Drawing for the job (mm, zero at the part's lowest x, y, z). Coordinates: 2 decimals unless noted, no trailing zeros. Loops run counter-clockwise (first coordinate to the right, second up) from the corner with the lowest first, then second, coordinate; pieces in that order, holes last. Notation, with made-up numbers: (1.5, 2) - (59.5, 2) arc R18 cw to (59.5, 21) - close; hole circle Ø11 at (22.25, 38). An arc over 180 degrees is marked (long way). One line per item, written item: value.
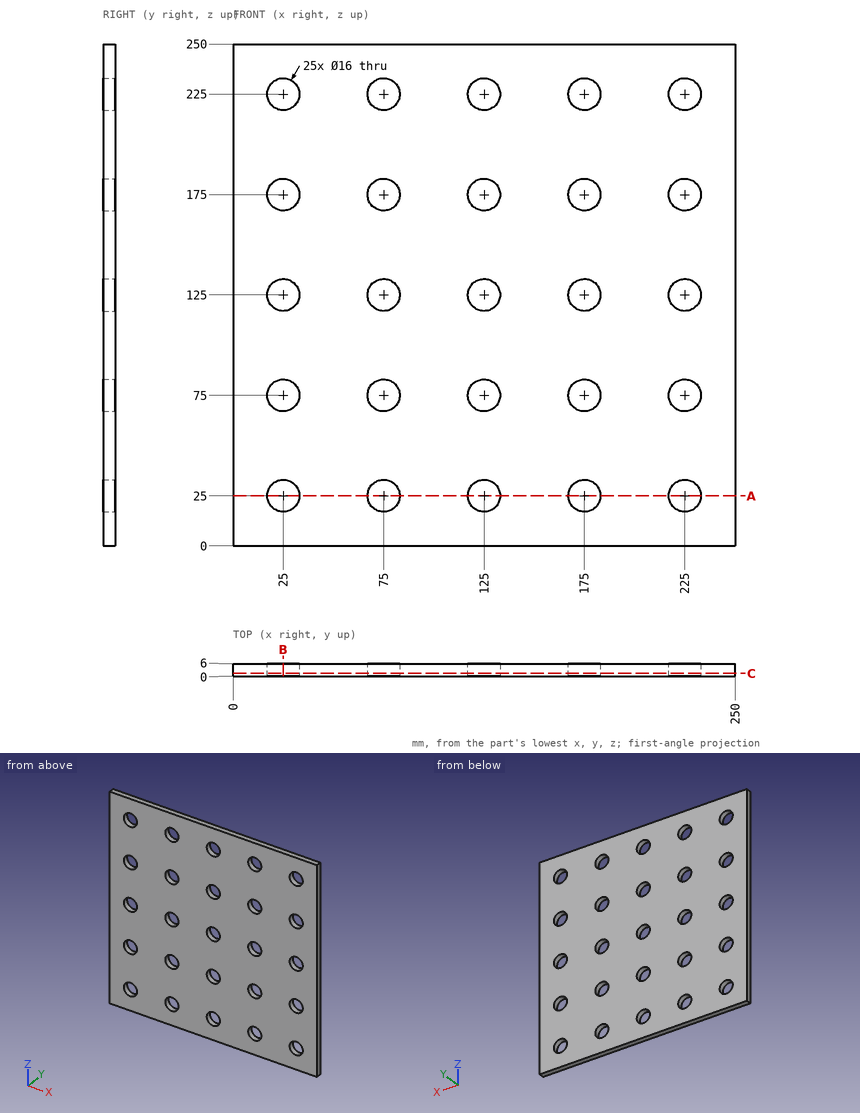
Item 1: Cut at B-B, the plane x = 25. Write the cut outline in (y, z), then the cut area to 3 significant figures.
Check result:
outline: (0, 0) - (6, 0) - (6, 17) - (0, 17) - close; (0, 33) - (6, 33) - (6, 67) - (0, 67) - close; (0, 83) - (6, 83) - (6, 117) - (0, 117) - close; (0, 133) - (6, 133) - (6, 167) - (0, 167) - close; (0, 183) - (6, 183) - (6, 217) - (0, 217) - close; (0, 233) - (6, 233) - (6, 250) - (0, 250) - close
area: 1,020 mm^2
Item 2: Cut at C-C, the plane y = 1.3. Give the number of separate pieces and of enclosed holes in the cut face, then the cut area to 3 significant figures.
Check result:
separate pieces: 1
enclosed holes: 25
area: 57,500 mm^2
Item 3: Probe probe 1 along Z at (x, y) = (225, 2.9); probe 2 along Z at (x, y) = (81.5, 1). List the from-to ranges inside material, lowest first. Write a range as from..to.
Check result:
probe 1: z = 0..17, 33..67, 83..117, 133..167, 183..217, 233..250
probe 2: z = 0..20.34, 29.66..70.34, 79.66..120.34, 129.66..170.34, 179.66..220.34, 229.66..250
Item 4: Cut at A-A, the plane z = 25. Write the cut outline in (x, y).
Check result:
outline: (0, 0) - (17, 0) - (17, 6) - (0, 6) - close; (33, 0) - (67, 0) - (67, 6) - (33, 6) - close; (83, 0) - (117, 0) - (117, 6) - (83, 6) - close; (133, 0) - (167, 0) - (167, 6) - (133, 6) - close; (183, 0) - (217, 0) - (217, 6) - (183, 6) - close; (233, 0) - (250, 0) - (250, 6) - (233, 6) - close
